Verification items for the finished model (mm, model axes). A direction names the side the tool comes from. Coordinates: 2 decimals unless noted, no trailing zeros. Order: outer loops, then holes, each group sorted by start corner. A loop starts at its lowest first (then second) coordinate and runs counter-clockwise, first axis right, second up. Notation, with made-up numbers: M 78,22 L 93,22 A35 ccw 93,61 Z; hole C 61.5,-7.5 d5. An arc over 180 degrees is marked long. Return JSON: item names as keys, results as strings. Group by question number.
1. Section check B-B, the plane z = -8.75. Record the cut outline in (x, y), plus the area to 3 significant figures.
2. Section check C-C, the plane x = -10.75. Record the cut outline in (y, z), plus the area to 3 significant figures.
3. Set-up check for faces 5 (the flat face through (1.4, -1.4, -10.4)), 6 (the flat face through (-7.24, 1.56, -1.07)): record each of +Z, -Z, +X, -X, +Y, -Y from which the full face is reachable in a straight line by a thin tool's end or side.
4. Material ranges on line 1 along Z through (x, y) = (-9.5, 0); line 2 along X through (y, z) = (1.25, -7), recorded low to high.
5. Mould release check, pull along X, two halves, no side actions. Record for faces 1 (the flat face through (1.07, 1.56, -7.24)), 2 (the flat face through (-10.4, -1.4, -1.4)), 3 (the cylindrical face through (2.19, 0.98, -8.06)), 4 (the cylindrical face through (-9.977, -3.434, 1.081)): +X half, -X half, draft (parallel to the pull), parting line (faces both ways), or undercut.
6. Gauge pin test, flat ends, axial feed: pin 1 (0.7 mm diameter, centred on x = -8.5, y = -2, fed in from +Z); pin 2 (0.5 mm diameter, centred on x = 2, z = -7, fed in from +Y); pin 3 (0.7 mm diameter, centred on x = -7, y = 2, fed in from -Z). Record the tip position at first contact, or that the pin passes through.
7. Section check A-A, the plane y = 0. Record the cut outline in (x, z), plus the area to 3 significant figures.
Autodesk Inventor part; units mm, degrees
ref_plane "Work Plane1" through (-12, 0, 0) normal (-1, 0, 0) x (0, -1, 0)
ref_plane "YZ Plane" through (0, 0, 0) normal (1, 0, 0) x (0, 1, 0)
ref_plane "XZ Plane" through (0, 0, 0) normal (0, 1, 0) x (-1, 0, 0)
sketch "Sketch2" plane through (0, 0, 0) normal (0, 1, 0) x (-1, 0, 0)
  line L0 (0, -12) -> (0, -8)
  arc A0 (8, 0) -> (0, -8) centre (8, -8) ccw
  line L1 (8, 0) -> (12, 0)
  point P0 (0, 0)
  dimension "d0" = 4
  dimension "d1" = 8
ref_plane "Work Plane1" through (-12, 0, 0) normal (-1, 0, 0) x (0, -1, 0)
sketch "Sketch3" plane through (-12, 0, 0) normal (-1, 0, 0) x (0, -1, 0)
  circle A0 centre (0, 0) radius 3.6
  circle A1 centre (0, 0) radius 2.4
  line L0 (-2.2627, 0.8) -> (-1.6217, 0.8)
  arc A2 (-1.6217, 0.8) -> (-0.9998, 0.9998) centre (-1.6217, 1.8675) ccw
  line L1 (-0.8, 2.2627) -> (-0.8, 1.6217)
  arc A3 (-0.9998, 0.9998) -> (-0.8, 1.6217) centre (-1.8675, 1.6217) ccw
  line L2 (2.2627, -0.8) -> (1.6217, -0.8)
  arc A4 (1.6217, -0.8) -> (0.9998, -0.9998) centre (1.6217, -1.8675) ccw
  line L3 (0.8, -2.2627) -> (0.8, -1.6217)
  arc A5 (0.9998, -0.9998) -> (0.8, -1.6217) centre (1.8675, -1.6217) ccw
  line L4 (0.9998, -0.9998) -> (-0.9998, 0.9998) construction
  line L5 (-2.1108, -1.1421) -> (-1, -1)
  line L6 (-1, -1) -> (-1.1421, -2.1108)
  line L7 (2.1108, 1.1421) -> (1, 1)
  line L8 (1, 1) -> (1.1421, 2.1108)
  line L9 (-1, -1) -> (1, 1) construction
  point P0 (0, 0)
  dimension "d3" = 4.8
  dimension "d2" = 7.2
  dimension "d4" = 45
  dimension "d5" = 1.6
  dimension "d6" = 0.641
  dimension "d7" = 2.828
  dimension "d8" = 2
  dimension "d9" = 1.37
sweep "Sweep1" add profiles "Sketch3" path "Sketch2" contours A0 | A1 L2 A4 A5 L3 L6 L5 L0 A2 A3 L1 L8 L7 | L7 L8 A1 | A1 L3 A5 A4 L2 | L1 A3 A2 L0 A1 | A1 L5 L6
extrude "Extrusion1" cut sketch "Sketch3" against normal blind 8 contours A1 L2 A4 A5 L3 L6 L5 L0 A2 A3 L1 L8 L7
extrude "Extrusion2" cut sketch "Sketch3" against normal blind 1.6 contours L7 L8 A1 | A1 L3 A5 A4 L2 | L1 A3 A2 L0 A1 | A1 L5 L6
pattern_circular "Circular Pattern1" count 2 over 90 about axis through (0, -10, 0) along (0, -1, 0) of "Extrusion1", "Extrusion2"
fillet "Fillet1" radius 0.1 2 edges at (-12, 3.6, 0) (0, 3.6, -12)
equation "\"d0\" = 0.5 * lu"
equation "\"d1\" = lu"
equation "\"d3\" = kd"
equation "\"d2\" = tlad"
equation "\"d5\" = axlet"
equation "\"d12\" = lu"
equation "\"d14\" = wall"
equation "\"d19\" = lf"
properties part number "25214-LtBluishGray" material "ABS Plastic"
Answers follow:
{
 "1": {"outline": "C 0,0 d7.2; hole M -2.26,0.8 A2.4 ccw -2.11,-1.14 L -1,-1 L -1.14,-2.11 A2.4 ccw 0.8,-2.26 L 0.8,-1.62 A1.07 cw 1,-1 A1.07 cw 1.62,-0.8 L 2.26,-0.8 A2.4 ccw 2.11,1.14 L 1,1 L 1.14,2.11 A2.4 ccw -0.8,2.26 L -0.8,1.62 A1.07 cw -1,1 A1.07 cw -1.62,0.8 Z", "area": "26.6 mm^2"},
 "2": {"outline": "C 0,0 d7.2; hole C 0,0 d4.8", "area": "22.6 mm^2"},
 "3": {"face 5": "-Z", "face 6": "-X"},
 "4": {"line 1": "-3.6 to -2.4, 2.4 to 3.6", "line 2": "-3.49 to -0.87, 1.03 to 3.33"},
 "5": {"face 1": "undercut", "face 2": "-X half", "face 3": "undercut", "face 4": "draft"},
 "6": {"pin 1": "z = 3.2", "pin 2": "y = 3.12", "pin 3": "z = -3.32"},
 "7": {"outline": "M -12,-3.5 A0.1 ccw -11.9,-3.6 L -8,-3.6 A4.4 cw -3.6,-8 L -3.6,-11.9 A0.1 ccw -3.5,-12 L -2.4,-12 L -2.4,-4 L 2.4,-4 L 2.4,-12 L 3.5,-12 A0.1 ccw 3.6,-11.9 L 3.6,-8 A11.6 ccw -8,3.6 L -11.9,3.6 A0.1 ccw -12,3.5 L -12,2.4 L -4,2.4 L -4,-2.4 L -12,-2.4 Z", "area": "71.3 mm^2"}
}
